Source: CAD feature listing. Evaluate the final solid. Frame: model axes, mm. A direction names the side the tool comes from. Give positions to 0.01 mm unless a question says otherwise; leave off trailing zeros. Order: outer loops, then holes, each group sorted by start corner. A loop starts at its lowest first (then second) coordinate and runs counter-clockwise, first axis right, second up.
1) Draft query along Y for faces 1 (the face through (-0.283, 22.156, 2.465)), 2 (the face through (-0.048, -2.465, 7.826)), 3 (the face through (0, 25, 2)). Return one class per face: released by +Y, released by -Y, zero draft, split by the parting line, or undercut.
2) Section C-C, the plane y = 19. Return loops of the section in (x, z).
3) Section D-D, the plane x = 3.5. Return loops of the section in (y, z), plus the area to 3 significant figures.
4) Material intervals for line 1 (Y direction, x = 0, z = 2.9) (3 decimals); line 2 (Z direction, x = -3.25, y = 10); line 3 (Y direction, x = 4.5, z = 22.5), sorted ascending.
5) Section B-B, the plane x = 0. Return loops of the section in (y, z) (3 decimals).
6) Section A-A, the plane z = 13. Return loops of the section in (x, y) (3 decimals), plus the area to 4 significant figures.
7) Access query for faces 4 (the face through (0.048, -2.465, 37.174)), 5 (the face through (0, 14, 5)), 6 (the face through (0, 7, 0)). Directions: +Z, -Z, +X, -X, +Y, -Y. A direction counts if a zero-diameter tool reaches every point of the face in a straight line with its end or side. Return the directions, or none.
8) First-contact query: P1, Ø5, axis at x = 0, y = 20, coming from the +Z side. Flat tip, straight axial feed; report the tip coordinate or a pass-through.
```python
from build123d import *

# Parameters (mm, degrees)
SKETCH_R     = 2.175
PAD_DEPTH    = 5
PAD001_DEPTH = 5
FILLET_R     = 2


with BuildPart() as part:
    # Sketch → Pad (new body)
    with BuildSketch(Plane.XY):
        with BuildLine():
            Line((-6.25, 0), (6.25, 0))
            Line((4.990412, 20.309504), (6.25, 0))
            ThreePointArc((4.990412, 20.309504), (0, 25), (-4.990412, 20.309504))
            Line((-4.990412, 20.309504), (-6.25, 0))
        make_face()
        with Locations((0, 20)):
            Circle(SKETCH_R, mode=Mode.SUBTRACT)
        with Locations((0, 10)):
            Circle(SKETCH_R, mode=Mode.SUBTRACT)
    extrude(amount=PAD_DEPTH)

    # Sketch001 (on Face3 of Pad) → Pad001 (join)
    with BuildSketch(Plane.XZ):
        with BuildLine():
            Line((6.25, 5), (6.25, 35))
            ThreePointArc((6.25, 35), (0, 41.25), (-6.25, 35))
            Line((-6.25, 5), (-6.25, 35))
            Line((-6.25, 5), (-6.25, 0))
            Line((-6.25, 0), (6.25, 0))
            Line((6.25, 0), (6.25, 5))
        make_face()
        with BuildLine():
            ThreePointArc((2.175, 35), (1.8e-05, 37.175), (-2.175, 35.000036))
            Line((-2.175, 10), (-2.175, 35.000036))
            ThreePointArc((-2.175, 10), (0, 7.825), (2.175, 10))
            Line((2.175, 35), (2.175, 10))
        make_face(mode=Mode.SUBTRACT)
    extrude(amount=PAD001_DEPTH)

    # Fillet
    fillet_edges = [part.edges().sort_by_distance(p)[0] for p in [
        (0, 0, 5),
    ]]
    fillet(fillet_edges, radius=FILLET_R)


solid = part.part
```
From the geometry:
1. face 1: undercut
1. face 2: zero draft
1. face 3: released by +Y
2. outline: (-5.07, 0) - (-1.93, 0) - (-1.93, 5) - (-5.07, 5) - close; (1.93, 0) - (5.07, 0) - (5.07, 5) - (1.93, 5) - close
3. outline: (-5, 0) - (23.57, 0) - (23.57, 5) - (2, 5) arc R2 cw to (0, 7) - (0, 40.18) - (-5, 40.18) - close
3. area: 320 mm2
4. line 1: y = -5 to 7.825, 12.175 to 17.825, 22.175 to 25
4. line 2: z = 0 to 5
4. line 3: y = -5 to 0
5. outline: (-5, 0) - (7.825, 0) - (7.825, 5) - (2, 5) arc R2 cw to (0, 7) - (0, 7.825) - (-5, 7.825) - close; (-5, 37.175) - (0, 37.175) - (0, 41.25) - (-5, 41.25) - close; (12.175, 0) - (17.825, 0) - (17.825, 5) - (12.175, 5) - close; (22.175, 0) - (25, 0) - (25, 5) - (22.175, 5) - close
6. outline: (-6.25, -5) - (-2.175, -5) - (-2.175, 0) - (-6.25, 0) - close; (2.175, -5) - (6.25, -5) - (6.25, 0) - (2.175, 0) - close
6. area: 40.75 mm2
7. face 4: +Y, -Y
7. face 5: +Z, +X, -X, +Y
7. face 6: -Z, +X, -X, +Y, -Y
8. P1: stops at z = 5
